Here's the drawing with two shaded views (mm, measured from the low corner). I have some questions. A direction names the side the tool comes from. Coordinates: 2 decimals unless noted, no trailing zeros. Write each loop counter-clockwise with the first axis right and the second up, starting at its lowest first coordinate (ties: lowest second). Pieces come first, ordered by that corner, then holes.
Item 1: Thinking about a two-plate mould opening in Z: for the marked faces 1, 2 and 3, which applies, +Z half, -Z half, draft (parallel to the pull), parting line (faces both ways), or undercut?
Item 2: Which directions (+Z, -Z, +X, -X, +Y, -Y) give clear straight access to the entire face, cutting with the end or side of a thin tool? Please do the marked faces 4, 5, 6, 7 and 8.
Item 3: For P1, Ø5, axis at x = 13, y = 17, coming from the +Z side; P2, Ø1, axis at x = 13.5, z = 3, coming from the +Y side; P3, Ø3.5, axis at y = 4, z = 5, coming from the -X side; P4, Ø1, axis at y = 4.5, z = 3, coming from the +X side (1 decimal), each with a flat end and sliding along its axis, tell me the tip position at first contact or that it passes through.
Item 4: I want a section at B-B on x = 10. Please give me the cut outline in (y, z).
Item 5: If I drill on probe 1 along Y at (x, z) = (10, 0.15); probe 2 along Z at (x, y) = (10, 1.4); probe 3 along X at (y, z) = (17, 0.4), over which ranges is the centre line in solid material (lowest first)?
Item 6: I want a section at C-C on x = 13. Please give me the cut outline in (y, z) (1 decimal).
Item 7: I want a section at A-A on y = 17. Please give me the cut outline in (x, z).
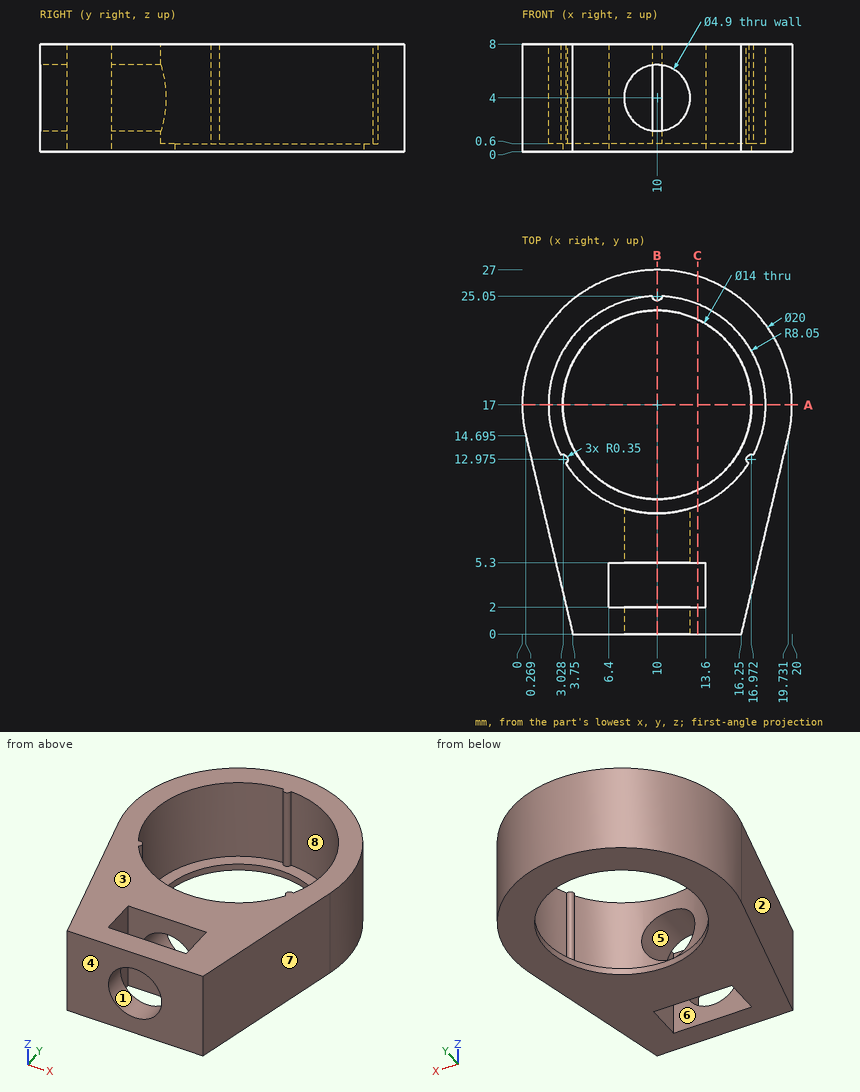
Response values:
1. face 1: undercut
1. face 2: draft
1. face 3: +Z half
2. face 4: +Z, -Z, +X, -X, -Y
2. face 5: -Y
2. face 6: +Z, -Z
2. face 7: +Z, -Z, +X, -Y
2. face 8: +Z
3. P1: passes through
3. P2: stops at y = 26.54
3. P3: stops at x = 2.39
3. P4: stops at x = 17.4
4. outline: (0, 0) - (2, 0) - (2, 1.55) - (0, 1.55) - close; (0, 6.45) - (2, 6.45) - (2, 8) - (0, 8) - close; (5.3, 0) - (10, 0) - (10, 0.6) - (8.95, 0.6) - (8.95, 1.55) - (5.3, 1.55) - close; (5.3, 6.45) - (8.95, 6.45) - (8.95, 8) - (5.3, 8) - close; (24, 0) - (27, 0) - (27, 8) - (24.7, 8) - (24.7, 0.6) - (24, 0.6) - close
5. probe 1: y = 0 to 2, 5.3 to 10, 24 to 27
5. probe 2: z = 0 to 1.55, 6.45 to 8
5. probe 3: x = 0 to 3, 17 to 20
6. outline: (0, 0) - (2, 0) - (2, 8) - (0, 8) - close; (5.3, 0) - (10.7, 0) - (10.7, 0.6) - (9.5, 0.6) - (9.5, 8) - (5.3, 8) - close; (23.3, 0) - (26.5, 0) - (26.5, 8) - (24.5, 8) - (24.5, 0.6) - (23.3, 0.6) - close
7. outline: (0, 0) - (3, 0) - (3, 0.6) - (1.95, 0.6) - (1.95, 8) - (0, 8) - close; (17, 0) - (20, 0) - (20, 8) - (18.05, 8) - (18.05, 0.6) - (17, 0.6) - close
